Design review of the part built by this model. Coordinates are the model's own, in mm. A direction names the side the tool comes from. Give positions to 0.01 mm unless a question says otherwise; leave off trailing zeros. Write each loop counter-clockwise with the first axis right and the second up, starting at its lowest first coordinate (ties: lowest second). Pieces come first, ordered by that corner, then holes.
Autodesk Inventor part; units mm, degrees
ref_plane "YZ Plane" through (0, 0, 0) normal (1, 0, 0) x (0, 1, 0)
ref_plane "XZ Plane" through (0, 0, 0) normal (0, 1, 0) x (-1, 0, 0)
ref_plane "XY Plane" through (0, 0, 0) normal (0, 0, 1) x (1, 0, 0)
sketch "Sketch1" plane through (0, 0, 0) normal (0, 1, 0) x (-1, 0, 0)
  circle A0 centre (12.7, 0) radius 31.75
  circle A1 centre (0, 0) radius 88.9
  circle A2 centre (0, 98.425) radius 9.525
  arc A3 (9.1574, 101.0457) -> (24.7665, 85.3805) centre (31.1351, 107.3355) ccw
  arc A4 (-24.7665, 85.3805) -> (-9.1574, 101.0457) centre (-31.1351, 107.3355) ccw
  circle A5 centre (-98.425, 0) radius 9.525
  circle A6 centre (0, -98.425) radius 9.525
  circle A7 centre (98.425, 0) radius 9.525
  arc A8 (85.3805, 24.7665) -> (101.0457, 9.1574) centre (107.3355, 31.1351) ccw
  arc A9 (24.7665, -85.3805) -> (9.1574, -101.0457) centre (31.1351, -107.3355) ccw
  arc A10 (-9.1574, -101.0457) -> (-24.7665, -85.3805) centre (-31.1351, -107.3355) ccw
  arc A11 (-85.3805, -24.7665) -> (-101.0457, -9.1574) centre (-107.3355, -31.1351) ccw
  arc A12 (-101.0457, 9.1574) -> (-85.3805, 24.7665) centre (-107.3355, 31.1351) ccw
  arc A13 (101.0457, -9.1574) -> (85.3805, -24.7665) centre (107.3355, -31.1351) ccw
  line L0 (98.425, 0) -> (88.9, 0)
  line L1 (0, 98.425) -> (0, 88.9)
  line L2 (0, -98.425) -> (0, -88.9)
  line L3 (-98.425, 0) -> (-88.9, 0)
  line L4 (12.7, 0) -> (0, 0)
  dimension "d20" = 177.8
  dimension "d0" = 63.5
  dimension "d2" = 19.05
  dimension "d3" = 22.86
  dimension "d21" = 12.7
extrude "Extrusion1" add sketch "Sketch1" along normal blind 6.35
sketch "Sketch3" plane through (0, 6.35, 0) normal (0, 1, 0) x (1, 0, 0)
  circle A0 centre (-12.7, 0) radius 31.75
  arc A1 (101.0457, -9.1574) -> (101.0457, 9.1574) centre (98.425, 0) ccw
  arc A2 (101.0457, -9.1574) -> (85.3805, -24.7665) centre (107.3355, -31.1351) ccw
  arc A3 (24.7665, -85.3805) -> (85.3805, -24.7665) centre (0, 0) ccw
  arc A4 (24.7665, -85.3805) -> (9.1574, -101.0457) centre (31.1351, -107.3355) ccw
  arc A5 (-9.1574, -101.0457) -> (9.1574, -101.0457) centre (0, -98.425) ccw
  arc A6 (-9.1574, -101.0457) -> (-24.7665, -85.3805) centre (-31.1351, -107.3355) ccw
  arc A7 (-85.3805, -24.7665) -> (-24.7665, -85.3805) centre (0, 0) ccw
  arc A8 (-85.3805, -24.7665) -> (-101.0457, -9.1574) centre (-107.3355, -31.1351) ccw
  arc A9 (-101.0457, 9.1574) -> (-101.0457, -9.1574) centre (-98.425, 0) ccw
  arc A10 (-101.0457, 9.1574) -> (-85.3805, 24.7665) centre (-107.3355, 31.1351) ccw
  arc A11 (-24.7665, 85.3805) -> (-85.3805, 24.7665) centre (0, 0) ccw
  arc A12 (-24.7665, 85.3805) -> (-9.1574, 101.0457) centre (-31.1351, 107.3355) ccw
  arc A13 (9.1574, 101.0457) -> (-9.1574, 101.0457) centre (0, 98.425) ccw
  arc A14 (9.1574, 101.0457) -> (24.7665, 85.3805) centre (31.1351, 107.3355) ccw
  arc A15 (85.3805, 24.7665) -> (24.7665, 85.3805) centre (0, 0) ccw
  arc A16 (85.3805, 24.7665) -> (101.0457, 9.1574) centre (107.3355, 31.1351) ccw
hole "Hole1" at (98.425, 6.35, 0) at (0, 6.35, 98.425) at (-98.425, 6.35, 0) at (0, 6.35, -98.425) direction (0, -1, 0) diameter 6.5278 depth 12.2936 tip angle 118
sketch "Sketch8" plane through (0, 6.35, 0) normal (0, 1, 0) x (1, 0, 0)
  circle A0 centre (-12.7, 0) radius 31.75
  circle A1 centre (-12.7, 0) radius 47.625
  line L0 (-12.7, 0) -> (-12.7, 47.625)
  point P0 (0, 0)
  point P1 (-53.9445, 23.8125)
  point P2 (-53.9445, -23.8125)
  point P3 (-12.7, -47.625)
  point P4 (28.5445, -23.8125)
  point P5 (28.5445, 23.8125)
  dimension "d38" = 95.25
  dimension "d41" = 360
hole "Hole3" at (-12.7, 6.35, -47.625) at (-53.9445, 6.35, -23.8125) at (-53.9445, 6.35, 23.8125) at (-12.7, 6.35, 47.625) at (28.5445, 6.35, 23.8125) at (28.5445, 6.35, -23.8125) direction (0, -1, 0) diameter 6.5278 end through all
sketch "Sketch9" plane through (0, 6.35, 0) normal (0, 1, 0) x (1, 0, 0)
  circle A0 centre (-12.7, 0) radius 31.75
  circle A1 centre (-12.7, 0) radius 63.5
  circle A2 centre (-12.7, 0) radius 82.55
  arc A3 (34.6487, 67.621) -> (23.7221, 52.0162) centre (29.1854, 59.8186) ccw
  arc A4 (23.7221, -52.0162) -> (34.6487, -67.621) centre (29.1854, -59.8186) ccw
  line L0 (0, 0) -> (50.8, 0)
  line L1 (-12.7, 0) -> (29.1854, 59.8186)
  line L2 (29.1854, -59.8186) -> (-12.7, 0)
  arc A5 (67.0372, -21.3655) -> (48.6363, -16.435) centre (57.8367, -18.9003) ccw
  arc A6 (48.6363, 16.435) -> (67.0372, 21.3655) centre (57.8367, 18.9003) ccw
  line L3 (-12.7, 0) -> (57.8367, 18.9003)
  line L4 (-12.7, 0) -> (57.8367, -18.9003)
  dimension "d50" = 31.75
  dimension "d51" = 19.05
  dimension "d52" = 55
  dimension "d53" = 55
  dimension "d54" = 40
  dimension "d55" = 40
extrude "Extrusion3" cut sketch "Sketch9" against normal blind 25.4 contours A1 A3 A2 A6 | A5 A2 A4 A1
sketch "Sketch10" plane through (0, 6.35, 0) normal (0, 1, 0) x (1, 0, 0)
  circle A0 centre (-98.425, 0) radius 3.2639
  line L0 (-12.7, 0) -> (-98.425, 0)
  arc A1 (-32.2465, 53.7034) -> (-62.1934, 28.575) centre (-12.7, 0) ccw
  arc A2 (-73.1919, 34.925) -> (-62.1934, 28.575) centre (-67.6926, 31.75) ccw
  arc A3 (-32.2465, 53.7034) -> (-36.5901, 65.6375) centre (-34.4183, 59.6705) ccw
  arc A4 (-36.5901, 65.6375) -> (-73.1919, 34.925) centre (-12.7, 0) ccw
  circle A5 centre (-98.425, 0) radius 3.2639
  circle A6 centre (-12.7, 0) radius 31.75
  arc A7 (-62.1934, -28.575) -> (-32.2465, -53.7034) centre (-12.7, 0) ccw
  arc A8 (-62.1934, -28.575) -> (-73.1919, -34.925) centre (-67.6926, -31.75) ccw
  arc A9 (-36.5901, -65.6375) -> (-32.2465, -53.7034) centre (-34.4183, -59.6705) ccw
  arc A10 (-73.1919, -34.925) -> (-36.5901, -65.6375) centre (-12.7, 0) ccw
  circle A11 centre (-12.7, 0) radius 31.75
  dimension "d58" = 114.3
  dimension "d59" = 12.7
  dimension "d60" = 70
  dimension "d61" = 30
extrude "Extrusion4" cut sketch "Sketch10" against normal blind 25.4 contours A1 A2 A4 A3 | A7 A9 A10 A8
properties part number "LargeBearingPlate" material "Aluminum 6061"
(1) Mouldability with a two-part tool opening along Z and no side actions: class faces 3 (the face through (-15.056, 3.131, 91.086)), 4 (the face through (-63.3, 3.13, -62.42)), 5 (the face through (-101.18, 3.13, 1.75)) as pulls with the +Z half, pulls with the -Z half, needs draft (parallel to the pull), parting line crosses it, or undercut.
Resolved:
face 3: pulls with the +Z half
face 4: pulls with the -Z half
face 5: undercut
(2) Consider section D-D, the plane y = 2.25. Give the number of separate pieces and of enclosed holes in the cut face, then the cut area to 3 significant figures.
Resolved:
separate pieces: 1
enclosed holes: 15
area: 19,100 mm2
(3) Clearance check with flat-ended pins moving along their axes: P1, Ø7.5, axis at x = 0, z = -98.425, coming from the +Y side; P2, Ø3, axis at x = 74, y = 1, coming from the +Z side; P3, Ø1, axis at y = 2, z = 36, coming from the -X side; P4, Ø2, axis at x = -11.5, y = 1, coming from the -Z side. State where each tip first meets the part, or that it passes through.
Resolved:
P1: stops at y = 6.35
P2: stops at z = 51.45
P3: stops at x = -81.5
P4: stops at z = -97.5
(4) Consider section A-A, the plane z = 0. Give the boundary of the cut face in (x, y), then the cut area to 3 significant figures.
Resolved:
outline: (-107.95, 0) - (-101.69, 0) - (-101.69, 6.35) - (-107.95, 6.35) - close; (-95.16, 0) - (-44.45, 0) - (-44.45, 6.35) - (-95.16, 6.35) - close; (19.05, 0) - (95.16, 0) - (95.16, 6.35) - (19.05, 6.35) - close; (101.69, 0) - (107.95, 0) - (107.95, 6.35) - (101.69, 6.35) - close
area: 885 mm2
(5) Consider section B-B, the plane x = 0. Give the boundary of the cut face in (y, z), then the cut area to 4 significant figures.
Resolved:
outline: (0, -107.95) - (6.35, -107.95) - (6.35, -101.69) - (0, -101.69) - close; (0, -95.16) - (6.35, -95.16) - (6.35, -29.1) - (0, -29.1) - close; (0, 29.1) - (6.35, 29.1) - (6.35, 95.16) - (0, 95.16) - close; (0, 101.69) - (6.35, 101.69) - (6.35, 107.95) - (0, 107.95) - close
area: 918.5 mm2
(6) To check wall thickness, follow L1, parallel to Z at x = -46.5, y = 3.75; L2, parallel to Z at x = 40.5, y = 2.25; L3, parallel to X at y = 3, z = -50. State the ranges of each line that lie inside material, in increasing order.
Resolved:
L1: z = -75.77 to -61.13, -46.08 to 46.08, 61.13 to 75.77
L2: z = -79.14 to -63.12, -34.67 to 34.67, 63.12 to 79.14
L3: x = -73.51 to -61.48, -40.38 to -14.94, -10.46 to 26.44, 52.98 to 73.51
(7) Tool access review of faces 1 (the face through (-57.337, 3.219, -53.727)), 2 (the face through (62.42, 3.13, -63.3)): name each direction out of +Z, -Z, +X, -X, +Y, -Y from which nothing blocks a thin tool from reaching the whole face with its end or side.
Resolved:
face 1: +Y, -Y
face 2: -Z, +X, +Y, -Y
(8) Consider section C-C, the plane x = 72. Give the boundary of the cut face in (y, z), then the cut area to 3 significant figures.
Resolved:
outline: (0, -52.15) - (6.35, -52.15) - (6.35, 52.15) - (0, 52.15) - close
area: 662 mm2
